from build123d import *

# Parameters (mm, degrees)
F0_W           = 203.2
F0_H           = 152.4
F1_DEPTH       = 101.6
F2_R           = 25.4
F3_R           = 25.4
F4_W           = 101.6
F4_H           = 76.2
F5_DEPTH       = 38.1
F7_DEPTH       = 25.4
F8_R           = 3.175
F9_DEPTH       = 12.7
F10_W          = 101.6
F10_H          = 25.457462908
F11_DEPTH      = 101.6
F11_DEPTH_BACK = 25.4
F12_R          = 38.1
F13_DEPTH      = 4.699
F15_W          = 152.4
F15_H          = 12.7
F16_DEPTH      = 6.35
F16_DEPTH_BACK = 6.35
F17_R          = 6.35
F18_DEPTH      = 19.05


with BuildPart() as f1:
    # F0 (on Front) → F1 (new body)
    with BuildSketch(Plane.XZ):
        Rectangle(F0_W, F0_H)
    extrude(amount=F1_DEPTH)

    # F2
    f2_edges = [f1.edges().sort_by_distance(p)[0] for p in [
        (101.6, -50.8, 76.2),
    ]]
    fillet(f2_edges, radius=F2_R)

    # F3
    f3_edges = [f1.edges().sort_by_distance(p)[0] for p in [
        (-101.6, -50.8, 76.2),
        (101.6, -50.8, -76.2),
        (-101.6, -50.8, -76.2),
    ]]
    fillet(f3_edges, radius=F3_R)

    # F4 (on face) → F5 (cut)
    with BuildSketch(Plane.XZ.offset(101.6)):
        Rectangle(F4_W, F4_H)
    extrude(amount=-F5_DEPTH, mode=Mode.SUBTRACT)

    # F6 (on face) → F7 (join)
    with BuildSketch(Plane.XZ.offset(63.5)):
        Polygon((-12.7, 19.05), (-25.4, 19.05), (-25.4, -19.05), (-25.4, -25.4), (25.4, -25.4), (25.4, -19.05), (25.4, 19.05), (12.7, 19.05), (12.7, -19.05), (-12.7, -19.05), align=None)
    extrude(amount=F7_DEPTH)

    # F8 (on face) → F9 (cut)
    with BuildSketch(Plane.XY.offset(-19.05)):
        with Locations((0, -76.2)):
            Circle(F8_R)
    extrude(amount=-F9_DEPTH, mode=Mode.SUBTRACT)

    # F10 (on face) → F11 (join, two sides)
    with BuildSketch(Plane.YZ.offset(101.6)) as f11_sk:
        with Locations((-50.8, -63.528731454)):
            Rectangle(F10_W, F10_H)
    extrude(amount=F11_DEPTH)
    extrude(f11_sk.sketch, amount=-F11_DEPTH_BACK)

    # F12 (on face) → F13 (cut)
    with BuildSketch(Plane.XY.offset(-50.8)):
        with Locations((152.4, -50.8)):
            Circle(F12_R)
    extrude(amount=-F13_DEPTH, mode=Mode.SUBTRACT)

    # F15 (on offset) → F16 (join, two sides)
    with BuildSketch(Plane(origin=(0, -50.8, 0), x_dir=(-1, 0, 0), z_dir=(0, 1, 0))) as f16_sk:
        with Locations((-76.2, 69.85)):
            Rectangle(F15_W, F15_H)
    extrude(amount=F16_DEPTH)
    extrude(f16_sk.sketch, amount=-F16_DEPTH_BACK)

    # F17 (on face) → F18 (join)
    with BuildSketch(Plane.XY.offset(76.2)):
        with Locations((152.4, -50.8)):
            Circle(F17_R)
    extrude(amount=-F18_DEPTH)


solid = f1.part
Input: part model. Units: mm. Frame: model coordinates. A direction names the side the tool comes from. Coordinates: 2 decimals unless noted, no trailing zeros. Order: outer loops, then holes, each group sorted by start corner. A loop starts at its lowest first (then second) coordinate and runs counter-clockwise, first axis right, second up.
1. Cut plane B-B, the plane x = 0. Return loops of the section in (y, z) (3 decimals).
Checked values:
outline: (-101.6, -76.2) - (0, -76.2) - (0, 76.2) - (-101.6, 76.2) - (-101.6, 38.1) - (-63.5, 38.1) - (-63.5, -19.05) - (-73.025, -19.05) - (-73.025, -25.4) - (-63.5, -25.4) - (-63.5, -38.1) - (-101.6, -38.1) - close; (-88.9, -25.4) - (-79.375, -25.4) - (-79.375, -19.05) - (-88.9, -19.05) - close
2. Access query for faces 1 (the flat face through (152, -51, 57.15)), 2 (the flat face through (-101.6, -50, -1)), 3 (the flat face through (-50.8, -83, -1)). Directions: +Z, -Z, +X, -X, +Y, -Y. A direction counts if a zero-diameter tool reaches every point of the face in a straight line with its end or side. Return the directions, or none.
Checked values:
face 1: +X, +Y, -Y
face 2: +Z, -Z, -X, +Y, -Y
face 3: -Y
3. Cut plane C-C, the plane z = -30.5. Return loops of the section in (x, y), plus the area to 3 significant figures.
Checked values:
outline: (-101.6, -101.6) - (-50.8, -101.6) - (-50.8, -63.5) - (50.8, -63.5) - (50.8, -101.6) - (101.6, -101.6) - (101.6, 0) - (-101.6, 0) - close
area: 16,800 mm2
4. Cut plane D-D, the plane y = -50.8. Return loops of the section in (x, z).
Checked values:
outline: (-101.6, -50.8) arc R25.4 ccw to (-76.2, -76.2) - (76.2, -76.2) - (76.2, -76.26) - (203.2, -76.26) - (203.2, -50.8) - (190.5, -50.8) - (190.5, -55.5) - (114.3, -55.5) - (114.3, -50.8) - (101.6, -50.8) - (101.6, 50.8) arc R25.4 ccw to (98.2, 63.5) - (146.05, 63.5) - (146.05, 57.15) - (158.75, 57.15) - (158.75, 76.2) - (-76.2, 76.2) arc R25.4 ccw to (-101.6, 50.8) - close
5. Cut plane A-A, the plane y = -76.2. Count the separate pieces of the cut face and the enclosed holes in it, plus the area to 3 significant figures.
Checked values:
separate pieces: 3
enclosed holes: 1
area: 26,400 mm2
6. Draft query along X for faces 4 (the flat face through (123, -44.45, 70)), 5 (the flat face through (120, -51, 63.5)), 6 (the flat face through (101.6, -50, -1)), 7 (the flat face through (12.7, -76, 0)). Return one class per face: +X half, -X half, draft (parallel to the pull), parting line (faces both ways), or undercut.
Checked values:
face 4: draft
face 5: undercut
face 6: +X half
face 7: undercut
7. Ray query, line 1 along X through (y, z) = (-80.5, -18); line 2 along Z through (x, y) = (18.5, -67); line 3 along X through (y, z) = (-76, -22). Return the intervals inside material, ascending.
Checked values:
line 1: x = -101.6 to -50.8, -25.4 to -12.7, 12.7 to 25.4, 50.8 to 101.6
line 2: z = -76.2 to -38.1, -25.4 to 19.05, 38.1 to 76.2
line 3: x = -101.6 to -50.8, -25.4 to -3.17, 3.17 to 25.4, 50.8 to 101.6
8. Contact query for flat-ended pins moving along their axis: P1, Ø6, axis at x = 20.5, y = -21.5, coming from the -Z side; P2, Ø19, axis at y = -88, z = -11.5, coming from the +X side; P3, Ø8, axis at x = -32, z = 25.5, coming from the -Y side. Output: stop coordinate, or through.
Checked values:
P1: stops at z = -76.2
P2: stops at x = 101.6
P3: stops at y = -63.5
